Here's how the part is built. I have some questions about the finished solid (model axes, mm). Give positions to 0.01 mm unless a question says otherwise; leave off trailing zeros. Write each loop counter-clockwise with the first axis right and the second up, starting at its lowest first coordinate (ties: lowest second). Pieces come first, ordered by that corner, then holes. Notation, with made-up numbers: (29.25, 29) -> (39.25, 29) arc R22 cw to (39.25, 40) -> close; hole circle Ø8 at (68.25, 6.5). An arc over 180 degrees is marked (long way). Put each result on its own line as item: value. Start each with the question number.
from build123d import *

# Parameters (mm, degrees)
SKETCH1_R           = 2.25
SKETCH1_R_2         = 1.5
SKETCH1_W           = 20
SKETCH1_H           = 40.5
BOSS_EXTRUDE1_DEPTH = 3


with BuildPart() as part:
    # Sketch1 → Boss-Extrude1 (new body)
    with BuildSketch(Plane.XY):
        with BuildLine():
            Line((-5, 44.75), (-5, -4.25))
            Line((-5, -4.25), (5.287636044, -85.486762889))
            ThreePointArc((5.287636044, -85.486762889), (10, -89.64), (14.712363956, -85.486762889))
            Line((14.712363956, -85.486762889), (25, -4.25))
            Line((25, -4.25), (25, 44.75))
            ThreePointArc((25, 44.75), (10, 59.75), (-5, 44.75))
        make_face()
        with Locations((14.75, -4.25)):
            Circle(SKETCH1_R, mode=Mode.SUBTRACT)
        with Locations((5.25, -4.25)):
            Circle(SKETCH1_R, mode=Mode.SUBTRACT)
        with Locations((14.75, 44.75)):
            Circle(SKETCH1_R, mode=Mode.SUBTRACT)
        with Locations((5.25, 44.75)):
            Circle(SKETCH1_R, mode=Mode.SUBTRACT)
        with Locations((10, 52.25)):
            Circle(SKETCH1_R_2, mode=Mode.SUBTRACT)
        with Locations((10, -11.75)):
            Circle(SKETCH1_R_2, mode=Mode.SUBTRACT)
        with Locations((10, 20.25)):
            Rectangle(SKETCH1_W, SKETCH1_H, mode=Mode.SUBTRACT)
    extrude(amount=BOSS_EXTRUDE1_DEPTH)


solid = part.part
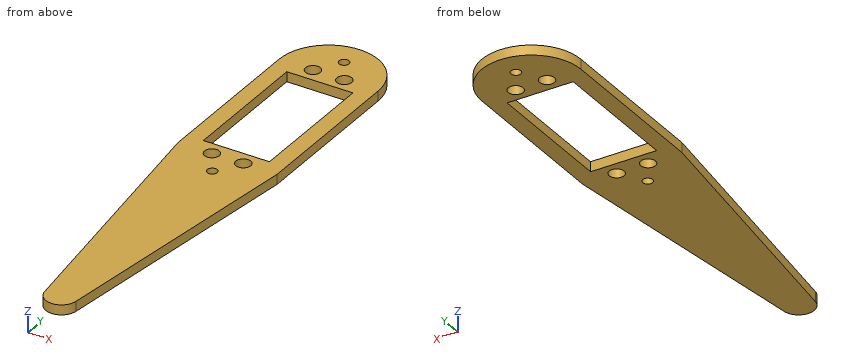
1) I want a section at A-A, the plane y = -11.75. Write out the boundary of the cut face in (x, z).
2) I want a section at B-B, the plane z = 1.55. Write out the boundary of the cut face in (x, y), and give its area (3 significant figures).
3) I'm going to push flat-ended pins straight in: pin 1 Ø4 at (x, y) = (5.25, 44.75) entering from +Z (3 decimals); pin 2 Ø0.9 at (x, z) = (8, 2) entering from +Y; pin 3 Ø1.5 at (y, z) = (-68.5, 2) entering from -X; pin 4 Ø0.9 at (x, z) = (14, 1) entering from -Y. Where does each tip first touch, or does it pass through?
4) I want a section at C-C, the plane y = 52.25. Write out the boundary of the cut face in (x, z).
5) I want a section at D-D, the plane x = -3. Write out the boundary of the cut face in (y, z), and give its area (3 significant figures).
6) I need wall thicknesses on probe 1 along Y at (x, z) = (10, 2.2); probe 2 along X at (y, z) = (8.5, 0.55); probe 3 along Y at (x, z) = (9, 1.7). Which ranges of each line are inside material? Lowest first, please.
Established:
1. outline: (-4.05, 0) -> (8.5, 0) -> (8.5, 3) -> (-4.05, 3) -> close; (11.5, 0) -> (24.05, 0) -> (24.05, 3) -> (11.5, 3) -> close
2. outline: (-5, -4.25) -> (5.29, -85.49) arc R4.75 ccw to (14.71, -85.49) -> (25, -4.25) -> (25, 44.75) arc R15 ccw to (-5, 44.75) -> close; hole (0, 0) -> (20, 0) -> (20, 40.5) -> (0, 40.5) -> close; hole circle Ø4.5 at (5.25, -4.25); hole circle Ø4.5 at (5.25, 44.75); hole circle Ø3 at (10, -11.75); hole circle Ø3 at (10, 52.25); hole circle Ø4.5 at (14.75, -4.25); hole circle Ø4.5 at (14.75, 44.75)
2. area: 2,570 mm2
3. pin 1: passes through
3. pin 2: stops at y = 59.67
3. pin 3: stops at x = 3.04
3. pin 4: stops at y = -88.05
4. outline: (-2.99, 0) -> (8.5, 0) -> (8.5, 3) -> (-2.99, 3) -> close; (11.5, 0) -> (22.99, 0) -> (22.99, 3) -> (11.5, 3) -> close
5. outline: (-20.04, 0) -> (52.23, 0) -> (52.23, 3) -> (-20.04, 3) -> close
5. area: 217 mm2
6. probe 1: y = -89.64 to -13.25, -10.25 to 0, 40.5 to 50.75, 53.75 to 59.75
6. probe 2: x = -5 to 0, 20 to 25
6. probe 3: y = -89.53 to -12.87, -10.63 to 0, 40.5 to 51.13, 53.37 to 59.72
